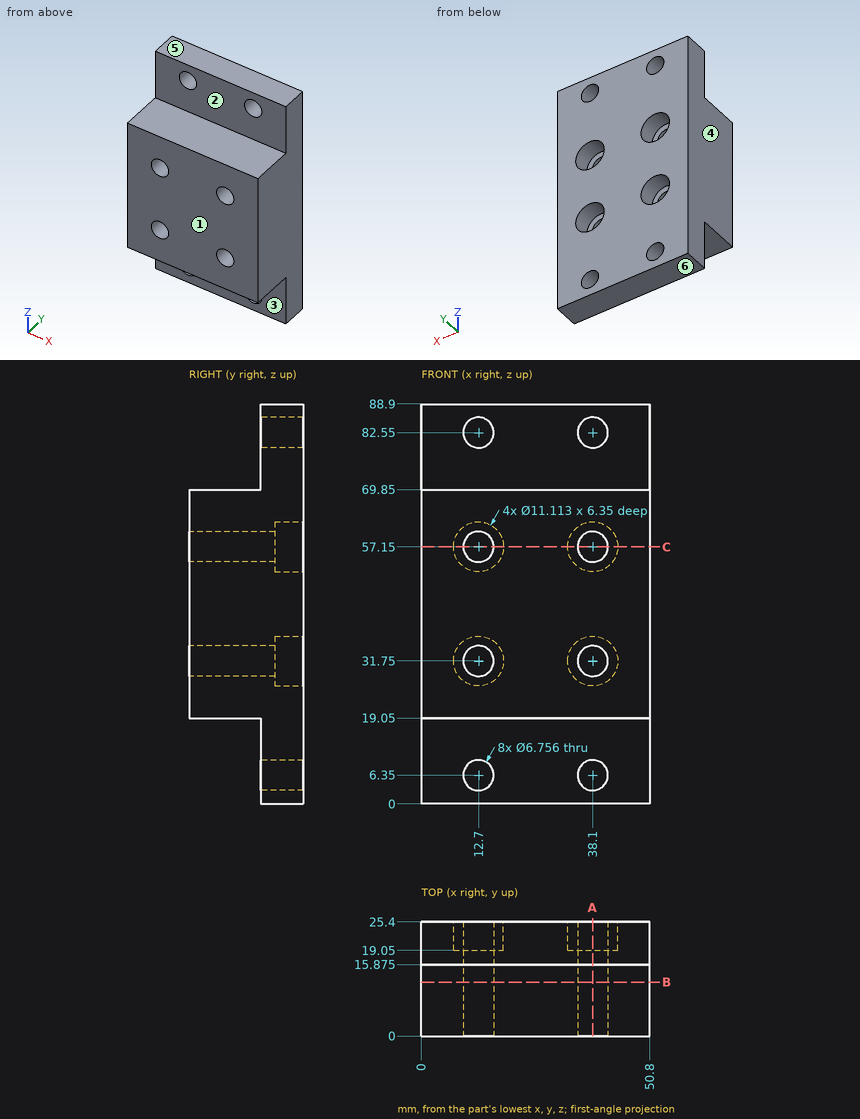
Source: three-view drawing plus pictorial views. Frame: mm from the lowest corner of the part. A direction names the side the tool comes from. Round coordinates to 2 decimals unless told otherwise and drop trailing zeros. Loops run counter-clockwise (first coordinate to the right, second up) from the corner with the lowest first, then second, coordinate; pieces in that order, holes last.
1. Section query A-A on x = 38.1. Give the number of separate pieces and of enclosed holes in the cut face, and give its area (3 significant figures).
2. Section query C-C on z = 57.15. Output: boundary loops of the cut face in (x, y).
3. Section query B-B on y = 12. Output: boundary loops of the cut face in (x, z), and give its area (3 significant figures).
4. Contact query for flat-ended pins moving along their axis: pin 1 (4 mm diameter, centred on x = 24, y = 19, fed in from -Z); pin 2 (8 mm diameter, centred on x = 30, y = 8, fed in from -Z); pin 3 (8 mm diameter, centred on x = 34, y = 4.5, fed in from +Z); pin 4 (10 mm diameter, centred on x = 12.7, z = 31.75, fed in from +Y). Output: stop coordinate, or through.
5. Ray query, L1, parallel to Z at x = 12.7, y = 12.5; L2, parallel to X at y = 20, z = 82.55; L3, parallel to Z at x = 38.1, y = 23. Return the intervals inside material, ascending.
6. Access query for the marked faces 1, 2 and 3. Directions: +Z, -Z, +X, -X, +Y, -Y. A direction counts if a zero-diameter tool reaches every point of the face in a straight line with its end or side. Return the directions, or none.
7. Mould query, pull axis Z, two halves, no side actions, for the marked faces 4, 5 and 6. Classes: released by +Z, released by -Z, zero draft, split by the parting line, or undercut.
Answers below:
1. separate pieces: 5
1. enclosed holes: 0
1. area: 1,130 mm2
2. outline: (0, 0) - (9.32, 0) - (9.32, 19.05) - (7.14, 19.05) - (7.14, 25.4) - (0, 25.4) - close; (16.08, 0) - (34.72, 0) - (34.72, 19.05) - (32.54, 19.05) - (32.54, 25.4) - (18.26, 25.4) - (18.26, 19.05) - (16.08, 19.05) - close; (41.48, 0) - (50.8, 0) - (50.8, 25.4) - (43.66, 25.4) - (43.66, 19.05) - (41.48, 19.05) - close
3. outline: (0, 19.05) - (50.8, 19.05) - (50.8, 69.85) - (0, 69.85) - close; hole circle Ø6.76 at (12.7, 31.75); hole circle Ø6.76 at (12.7, 57.15); hole circle Ø6.76 at (38.1, 31.75); hole circle Ø6.76 at (38.1, 57.15)
3. area: 2,440 mm2
4. pin 1: stops at z = 0
4. pin 2: stops at z = 19.05
4. pin 3: stops at z = 69.85
4. pin 4: stops at y = 19.05
5. L1: z = 19.05 to 28.37, 35.13 to 53.77, 60.53 to 69.85
5. L2: x = 0 to 9.32, 16.08 to 34.72, 41.48 to 50.8
5. L3: z = 0 to 2.97, 9.73 to 26.19, 37.31 to 51.59, 62.71 to 79.17, 85.93 to 88.9
6. face 1: +Z, -Z, +X, -X, -Y
6. face 2: +Z, +X, -X, -Y
6. face 3: -Z, +X, -X, -Y
7. face 4: zero draft
7. face 5: released by +Z
7. face 6: released by -Z
